Design review of the part built by this model. Coordinates are the model's own, in mm. Face numbers are marked on the shaded views. Coordinates: 2 decimals unless noted, no trailing zeros. Loops run counter-clockwise (first coordinate to the right, second up) from the corner with the lowest first, then second, coordinate; pieces in that order, holes last. Notation, with made-up numbers: (65, 61) -> (95, 61) arc R35 ccw to (95, 100) -> close; hole circle Ø7 at (-23, 89). An arc over 180 degrees is marked (long way). Answer as a JSON object with one key per item and string values.
```python
from build123d import *

# Parameters (mm, degrees)
F1_DEPTH = 12.7
F3_DEPTH = 5.08
F2_R     = 3.6923904974
F4_DEPTH = 12.701


with BuildPart() as f1:
    # F0 (on Top) → F1 (new body)
    with BuildSketch(Plane.XY):
        with BuildLine():
            Line((-54.1907071126, 81.808431102), (-61.2093408165, 56.2272694019))
            ThreePointArc((-61.2093408165, 56.2272694019), (-44.1142917545, -18.5841968693), (-36.5910920494, 57.7859390103))
            Line((-36.5910920494, 57.7859390103), (-44.0307071126, 81.808431102))
            Line((-44.0307071126, 81.808431102), (-54.1907071126, 81.808431102))
        make_face()
    extrude(amount=F1_DEPTH)

    # F2 (on face) → F3 (cut)
    with BuildSketch(Plane.XY.offset(12.7)):
        with BuildLine():
            ThreePointArc((-61.2093408165, 56.2272694019), (-68.2756243995, -12.0384858735), (-7.695419858, 20.2134059267))
            ThreePointArc((-7.695419858, 20.2134059267), (-15.7547342949, 43.9128527226), (-36.5910920494, 57.7859390103))
            ThreePointArc((-36.5910920494, 57.7859390103), (-49.0271224706, 59.0110087227), (-61.2093408165, 56.2272694019))
        make_face()
        with BuildLine():
            Line((-63.8565910506, 10.8681354841), (-62.1906724727, 10.8681354841))
            Line((-62.1906724727, 10.8681354841), (-62.1906724727, 3.817333427))
            add(Edge.make_bspline(
                [(-62.1906724727, 3.817333427), (-62.1906724727, 2.4877717429), (-61.5861820173, 1.8340970248)],
                knots=[0, 0, 0, 1, 1, 1], degree=2))
            add(Edge.make_bspline(
                [(-61.5861820173, 1.8340970248), (-60.9816915619, 1.1804223066), (-59.693381195, 1.1804223066)],
                knots=[0, 0, 0, 1, 1, 1], degree=2))
            add(Edge.make_bspline(
                [(-59.693381195, 1.1804223066), (-57.9862113, 1.1804223066), (-57.1992630956, 2.1117501211)],
                knots=[0, 0, 0, 1, 1, 1], degree=2))
            add(Edge.make_bspline(
                [(-57.1992630956, 2.1117501211), (-56.4123148912, 3.0430779355), (-56.4123148912, 5.1564146457)],
                knots=[0, 0, 0, 1, 1, 1], degree=2))
            Line((-56.4123148912, 5.1564146457), (-56.4123148912, 10.8681354841))
            Line((-56.4123148912, 10.8681354841), (-54.7654353828, 10.8681354841))
            Line((-54.7654353828, 10.8681354841), (-54.7654353828, 0))
            Line((-54.7654353828, 0), (-56.1235556711, 0))
            Line((-56.1235556711, 0), (-56.3615440393, 1.4564888138))
            Line((-56.3615440393, 1.4564888138), (-56.4503930302, 1.4564888138))
            add(Edge.make_bspline(
                [(-56.4503930302, 1.4564888138), (-56.9549283709, 0.6536747182), (-57.8529378138, 0.2268822444)],
                knots=[0, 0, 0, 1, 1, 1], degree=2))
            add(Edge.make_bspline(
                [(-57.8529378138, 0.2268822444), (-58.7509472567, -0.1999102293), (-59.9028109591, -0.1999102293)],
                knots=[0, 0, 0, 1, 1, 1], degree=2))
            add(Edge.make_bspline(
                [(-59.9028109591, -0.1999102293), (-61.8860473613, -0.1999102293), (-62.8713192059, 0.742523709)],
                knots=[0, 0, 0, 1, 1, 1], degree=2))
            add(Edge.make_bspline(
                [(-62.8713192059, 0.742523709), (-63.8565910506, 1.6849576473), (-63.8565910506, 3.7570430403)],
                knots=[0, 0, 0, 1, 1, 1], degree=2))
            Line((-63.8565910506, 3.7570430403), (-63.8565910506, 10.8681354841))
        make_face(mode=Mode.SUBTRACT)
        with BuildLine():
            Line((-42.1901300037, 0), (-43.8370095121, 0))
            Line((-43.8370095121, 0), (-43.8370095121, 7.0317629877))
            add(Edge.make_bspline(
                [(-43.8370095121, 7.0317629877), (-43.8370095121, 8.3581514935), (-44.4414999675, 9.0134128008)],
                knots=[0, 0, 0, 1, 1, 1], degree=2))
            add(Edge.make_bspline(
                [(-44.4414999675, 9.0134128008), (-45.0459904229, 9.668674108), (-46.337473968, 9.668674108)],
                knots=[0, 0, 0, 1, 1, 1], degree=2))
            add(Edge.make_bspline(
                [(-46.337473968, 9.668674108), (-48.0414706848, 9.668674108), (-48.8347652457, 8.7468658283)],
                knots=[0, 0, 0, 1, 1, 1], degree=2))
            add(Edge.make_bspline(
                [(-48.8347652457, 8.7468658283), (-49.6280598066, 7.8250575485), (-49.6280598066, 5.7022013036)],
                knots=[0, 0, 0, 1, 1, 1], degree=2))
            Line((-49.6280598066, 5.7022013036), (-49.6280598066, 0))
            Line((-49.6280598066, 0), (-51.274939315, 0))
            Line((-51.274939315, 0), (-51.274939315, 10.8681354841))
            Line((-51.274939315, 10.8681354841), (-49.9358580962, 10.8681354841))
            Line((-49.9358580962, 10.8681354841), (-49.6693111237, 9.3799148879))
            Line((-49.6693111237, 9.3799148879), (-49.5899816676, 9.3799148879))
            add(Edge.make_bspline(
                [(-49.5899816676, 9.3799148879), (-49.0822731487, 10.1827289835), (-48.1699844037, 10.6253873485)],
                knots=[0, 0, 0, 1, 1, 1], degree=2))
            add(Edge.make_bspline(
                [(-48.1699844037, 10.6253873485), (-47.2576956586, 11.0680457134), (-46.1375637387, 11.0680457134)],
                knots=[0, 0, 0, 1, 1, 1], degree=2))
            add(Edge.make_bspline(
                [(-46.1375637387, 11.0680457134), (-44.1733664059, 11.0680457134), (-43.1817482048, 10.1208520077)],
                knots=[0, 0, 0, 1, 1, 1], degree=2))
            add(Edge.make_bspline(
                [(-43.1817482048, 10.1208520077), (-42.1901300037, 9.1736583021), (-42.1901300037, 7.0888801961)],
                knots=[0, 0, 0, 1, 1, 1], degree=2))
            Line((-42.1901300037, 7.0888801961), (-42.1901300037, 0))
        make_face(mode=Mode.SUBTRACT)
        Polygon((-67.4676678917, 14.4982513947), (-67.4676678917, 0), (-69.152625539, 0), (-69.152625539, 6.8223332236), (-76.7904655712, 6.8223332236), (-76.7904655712, 0), (-78.4754232185, 0), (-78.4754232185, 14.4982513947), (-76.7904655712, 14.4982513947), (-76.7904655712, 8.3295928893), (-69.152625539, 8.3295928893), (-69.152625539, 14.4982513947), align=None, mode=Mode.SUBTRACT)
        with BuildLine():
            add(Edge.make_bspline(
                [(-25.1723750837, -0.0349049607), (-25.9498037533, -0.1999102293), (-27.0508966038, -0.1999102293)],
                knots=[0, 0, 0, 1, 1, 1], degree=2))
            add(Edge.make_bspline(
                [(-27.0508966038, -0.1999102293), (-29.4593388907, -0.1999102293), (-30.8539507287, 1.2692712974)],
                knots=[0, 0, 0, 1, 1, 1], degree=2))
            add(Edge.make_bspline(
                [(-30.8539507287, 1.2692712974), (-32.2485625667, 2.7384528242), (-32.2485625667, 5.3436321621)],
                knots=[0, 0, 0, 1, 1, 1], degree=2))
            add(Edge.make_bspline(
                [(-32.2485625667, 5.3436321621), (-32.2485625667, 7.974196926), (-30.9539058434, 9.5211213197)],
                knots=[0, 0, 0, 1, 1, 1], degree=2))
            add(Edge.make_bspline(
                [(-30.9539058434, 9.5211213197), (-29.65924912, 11.0680457134), (-27.4761024885, 11.0680457134)],
                knots=[0, 0, 0, 1, 1, 1], degree=2))
            add(Edge.make_bspline(
                [(-27.4761024885, 11.0680457134), (-25.4357488779, 11.0680457134), (-24.2458070366, 9.7242047273)],
                knots=[0, 0, 0, 1, 1, 1], degree=2))
            add(Edge.make_bspline(
                [(-24.2458070366, 9.7242047273), (-23.0558651952, 8.3803637412), (-23.0558651952, 6.1781780402)],
                knots=[0, 0, 0, 1, 1, 1], degree=2))
            Line((-23.0558651952, 6.1781780402), (-23.0558651952, 5.1373755763))
            Line((-23.0558651952, 5.1373755763), (-30.5413926717, 5.1373755763))
            add(Edge.make_bspline(
                [(-30.5413926717, 5.1373755763), (-30.4906218198, 3.2239490954), (-29.5735733074, 2.2323308943)],
                knots=[0, 0, 0, 1, 1, 1], degree=2))
            add(Edge.make_bspline(
                [(-29.5735733074, 2.2323308943), (-28.6565247951, 1.2407126932), (-26.9906062172, 1.2407126932)],
                knots=[0, 0, 0, 1, 1, 1], degree=2))
            add(Edge.make_bspline(
                [(-26.9906062172, 1.2407126932), (-25.2358386485, 1.2407126932), (-23.522322397, 1.9737168675)],
                knots=[0, 0, 0, 1, 1, 1], degree=2))
            Line((-23.522322397, 1.9737168675), (-23.522322397, 0.5045353407))
            add(Edge.make_bspline(
                [(-23.522322397, 0.5045353407), (-24.394946414, 0.130100308), (-25.1723750837, -0.0349049607)],
                knots=[0, 0, 0, 1, 1, 1], degree=2))
        make_face(mode=Mode.SUBTRACT)
        with BuildLine():
            add(Edge.make_bspline(
                [(-17.163273197, 10.4921138622), (-16.3096882495, 11.0680457134), (-15.2879248551, 11.0680457134)],
                knots=[0, 0, 0, 1, 1, 1], degree=2))
            add(Edge.make_bspline(
                [(-15.2879248551, 11.0680457134), (-14.5644402155, 11.0680457134), (-13.9900949535, 10.9474649402)],
                knots=[0, 0, 0, 1, 1, 1], degree=2))
            Line((-13.9900949535, 10.9474649402), (-14.218563787, 9.421166205))
            add(Edge.make_bspline(
                [(-14.218563787, 9.421166205), (-14.8912775746, 9.5703055825), (-15.4085056283, 9.5703055825)],
                knots=[0, 0, 0, 1, 1, 1], degree=2))
            add(Edge.make_bspline(
                [(-15.4085056283, 9.5703055825), (-16.7285477776, 9.5703055825), (-17.6646353595, 8.4993579253)],
                knots=[0, 0, 0, 1, 1, 1], degree=2))
            add(Edge.make_bspline(
                [(-17.6646353595, 8.4993579253), (-18.6007229413, 7.4284102681), (-18.6007229413, 5.8323016116)],
                knots=[0, 0, 0, 1, 1, 1], degree=2))
            Line((-18.6007229413, 5.8323016116), (-18.6007229413, 0))
            Line((-18.6007229413, 0), (-20.2476024497, 0))
            Line((-20.2476024497, 0), (-20.2476024497, 10.8681354841))
            Line((-20.2476024497, 10.8681354841), (-18.8894821615, 10.8681354841))
            Line((-18.8894821615, 10.8681354841), (-18.6990914669, 8.8563404777))
            Line((-18.6990914669, 8.8563404777), (-18.6197620108, 8.8563404777))
            add(Edge.make_bspline(
                [(-18.6197620108, 8.8563404777), (-18.0168581445, 9.916182011), (-17.163273197, 10.4921138622)],
                knots=[0, 0, 0, 1, 1, 1], degree=2))
        make_face(mode=Mode.SUBTRACT)
        with BuildLine():
            add(Edge.make_bspline(
                [(-36.5799508692, 1.6865442364), (-36.1134936674, 1.1613832371), (-35.301160037, 1.1613832371)],
                knots=[0, 0, 0, 1, 1, 1], degree=2))
            add(Edge.make_bspline(
                [(-35.301160037, 1.1613832371), (-34.8632614394, 1.1613832371), (-34.4570946242, 1.224846802)],
                knots=[0, 0, 0, 1, 1, 1], degree=2))
            add(Edge.make_bspline(
                [(-34.4570946242, 1.224846802), (-34.0509278091, 1.2883103669), (-33.8129394408, 1.3581202882)],
                knots=[0, 0, 0, 1, 1, 1], degree=2))
            Line((-33.8129394408, 1.3581202882), (-33.8129394408, 0.0983685256))
            add(Edge.make_bspline(
                [(-33.8129394408, 0.0983685256), (-34.0794864133, -0.0285586042), (-34.5998876452, -0.1142344168)],
                knots=[0, 0, 0, 1, 1, 1], degree=2))
            add(Edge.make_bspline(
                [(-34.5998876452, -0.1142344168), (-35.1202888771, -0.1999102293), (-35.5391484053, -0.1999102293)],
                knots=[0, 0, 0, 1, 1, 1], degree=2))
            add(Edge.make_bspline(
                [(-35.5391484053, -0.1999102293), (-38.6901144011, -0.1999102293), (-38.6901144011, 3.1224073916)],
                knots=[0, 0, 0, 1, 1, 1], degree=2))
            Line((-38.6901144011, 3.1224073916), (-38.6901144011, 9.589344652))
            Line((-38.6901144011, 9.589344652), (-40.2481449187, 9.589344652))
            Line((-40.2481449187, 9.589344652), (-40.2481449187, 10.3826392128))
            Line((-40.2481449187, 10.3826392128), (-38.6901144011, 11.0680457134))
            Line((-38.6901144011, 11.0680457134), (-37.998361544, 13.3876390095))
            Line((-37.998361544, 13.3876390095), (-37.046408071, 13.3876390095))
            Line((-37.046408071, 13.3876390095), (-37.046408071, 10.8681354841))
            Line((-37.046408071, 10.8681354841), (-33.8922688969, 10.8681354841))
            Line((-33.8922688969, 10.8681354841), (-33.8922688969, 9.589344652))
            Line((-33.8922688969, 9.589344652), (-37.046408071, 9.589344652))
            Line((-37.046408071, 9.589344652), (-37.046408071, 3.192217313))
            add(Edge.make_bspline(
                [(-37.046408071, 3.192217313), (-37.046408071, 2.2117052357), (-36.5799508692, 1.6865442364)],
                knots=[0, 0, 0, 1, 1, 1], degree=2))
        make_face(mode=Mode.SUBTRACT)
    extrude(amount=-F3_DEPTH, mode=Mode.SUBTRACT)

    # F2 (on face) → F4 (cut, through all)
    with BuildSketch(Plane.XY.offset(12.7)):
        with Locations((-49.1080991924, 74.8352557421)):
            Circle(F2_R)
    extrude(amount=-F4_DEPTH, mode=Mode.SUBTRACT)


solid = f1.part
```
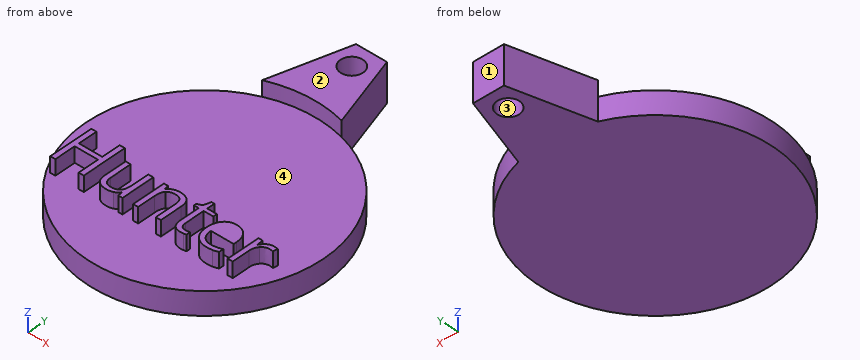
1) Add section B-B, the plane z = 9. Count the separate pieces of the cut face and the enclosed holes in it, and give its area (3 significant figures).
Completed:
{"separate pieces": "7", "enclosed holes": "1", "area": "619 mm²"}
2) Add section A-A, the plane z = 4. Give the boundary of the cut face in (x, y), and give its area (3 significant figures).
Completed:
{"outline": "(-61.21, 56.23) arc R38.88 ccw (long way) to (-36.59, 57.79) -> (-44.03, 81.81) -> (-54.19, 81.81) -> close; hole circle Ø7.38 at (-49.11, 74.84)", "area": "5,100 mm²"}
3) The part is to be moulded in two halves that separate along Y. For the marked faces 1, 2, 3 and 4, say which applies: pulls with the +Y half, pulls with the -Y half, needs draft (parallel to the pull), parting line crosses it, or undercut.
Completed:
{"face 1": "pulls with the +Y half", "face 2": "needs draft", "face 3": "undercut", "face 4": "undercut"}
4) Clearance check with flat-ended pins moving along their axes: pin 1 Ø1.5 at (y, z) = (10.5, 9.5) entering from +X; pin 2 Ø1.3 at (x, z) = (-68, 10) entering from +Y; pin 3 Ø2.5 at (y, z) = (7.5, 10) entering from +X (3 decimals). State where each tip first meets the part, or that it passes through.
Completed:
{"pin 1": "x = -13.99", "pin 2": "y = 14.5", "pin 3": "x = -17.425"}
5) Add section C-C, the plane y = 37. Give the boundary of the cut face in (x, z).
Completed:
{"outline": "(-81.63, 0) -> (-11.51, 0) -> (-11.51, 7.62) -> (-81.63, 7.62) -> close"}
6) Add section D-D, the plane y = 52. Give the boundary of the cut face in (x, z), and give its area (3 significant figures).
Completed:
{"outline": "(-68.95, 0) -> (-24.19, 0) -> (-24.19, 7.62) -> (-68.95, 7.62) -> close", "area": "341 mm²"}
7) Wall thickness on probe 1 along Z at (x, y) = (-51.5, 37); probe 2 along Y at (x, z) = (-46.5, 6.75); probe 3 along Y at (x, z) = (-64.5, 4.75): over which ranges is each line inside the solid? List them lowest first.
Completed:
{"probe 1": "0 to 7.62", "probe 2": "-18.66 to 72.22, 77.45 to 81.81", "probe 3": "-14.28 to 54.71"}
